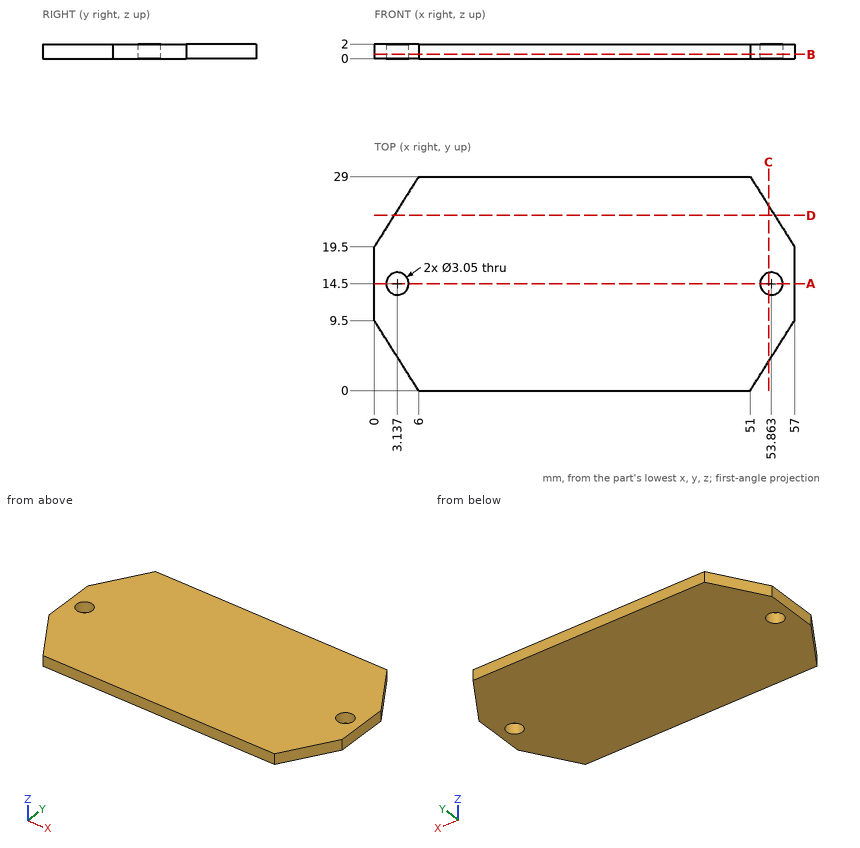
Input: dimensioned drawing with shaded views. Units: mm. Origin: part minimum x, y, z. Coordinates: 2 decimals unless noted, no trailing zeros. Write each loop counter-clockwise with the first axis right and the second up, starting at its lowest first coordinate (ties: lowest second). Pieces come first, ordered by that corner, then holes. Notation, with made-up numbers: M 80,1.25 L 135,1.25 A20 cw 135,6.25 Z; hole C 26.25,43.25 d8. An arc over 180 degrees is marked long. Answer as a JSON object with one key per item and string values. Group by question number.
(1) Section D-D on y = 23.75. Output: boundary loops of the cut face in (x, z).
(2) Section A-A on y = 14.5. Output: boundary loops of the cut face in (x, z), plus the area to 3 significant figures.
(3) Section B-B on z = 0.6. Give the number of separate pieces and of enclosed holes in the cut face, plus the area to 3 significant figures.
(4) Ray query, line 1 along X through (y, z) = (22.5, 1.1) (1 decimal); line 2 along X through (y, z) = (19.75, 1.65); line 3 along Y through (x, z) = (52, 0.4) (1 decimal). Return the intervals inside material, ascending. Write a range as [from, to].
(5) Section C-C on x = 53.5. Output: boundary loops of the cut face in (y, z).
Result set:
{
 "1": {"outline": "M 2.68,0 L 54.32,0 L 54.32,2 L 2.68,2 Z"},
 "2": {"outline": "M 0,0 L 1.61,0 L 1.61,2 L 0,2 Z; M 4.66,0 L 52.34,0 L 52.34,2 L 4.66,2 Z; M 55.39,0 L 57,0 L 57,2 L 55.39,2 Z", "area": "102 mm2"},
 "3": {"separate pieces": "1", "enclosed holes": "2", "area": "1,520 mm2"},
 "4": {"line 1": "x = [1.9, 55.1]", "line 2": "x = [0.16, 56.84]", "line 3": "y = [1.6, 27.4]"},
 "5": {"outline": "M 3.96,0 L 13.02,0 L 13.02,2 L 3.96,2 Z; M 15.98,0 L 25.04,0 L 25.04,2 L 15.98,2 Z"}
}
